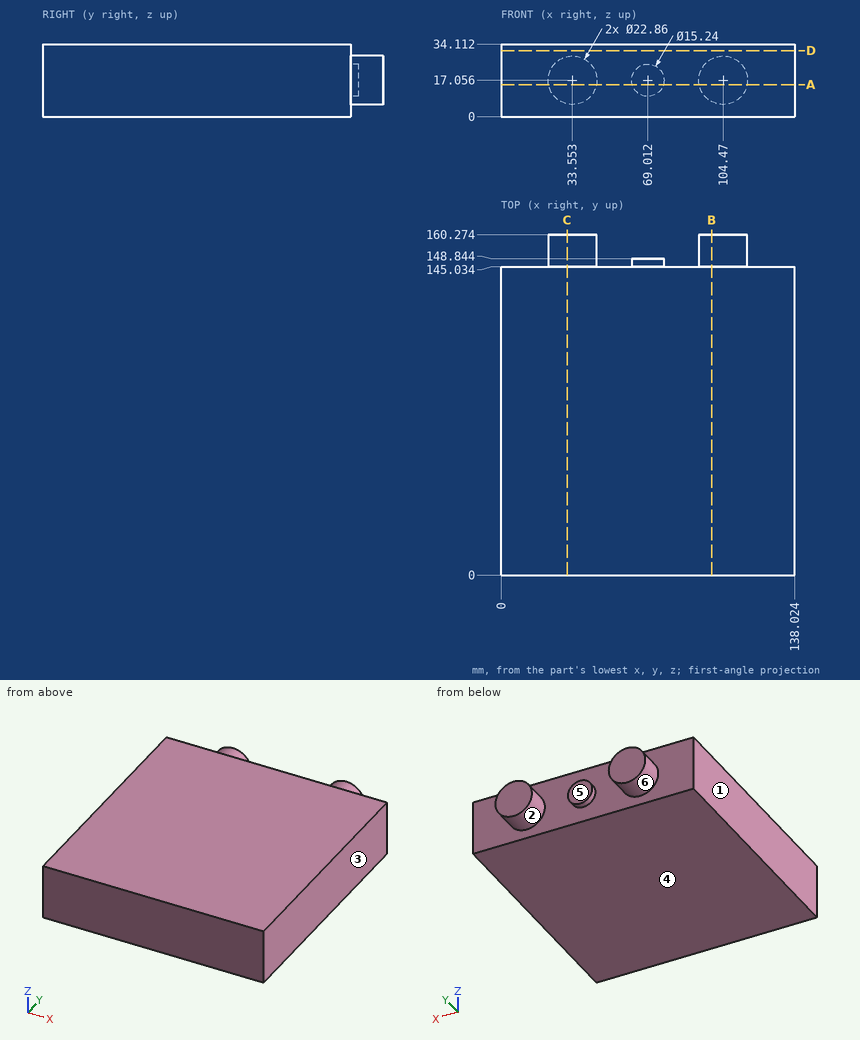
Could you check a few things on this drawing? It's one solid part, dimensions in mm from its lowest x, y, z. A direction names the side the tool comes from. Give positions to 0.01 mm unless a question says otherwise; leave off trailing zeros. Loops run counter-clockwise (first coordinate to the right, second up) from the corner with the lowest first, then second, coordinate; pieces in that order, holes last. Notation, with made-up numbers: M 49.5,-11.5 L 63.5,-11.5 A16 ccw 63.5,4.5 Z; hole C 79,-27.5 d10. An arc over 180 degrees is marked long. One line per question, with ' | ' between items. Start each with the question number.
Q1. If we section it at B-B (x = 99): Please give me the cut outline in (y, z).
Q2. If we section it at D-D (z = 31): Please give me the cut outline in (x, y).
Q3. If we mould it in two halves opening along X, with no side actions, what happens to the marked faces 1, 2 and 3? For each: +X half, -X half, draft (parallel to the pull), parting line (faces both ways), or undercut.
Q4. For the marked faces 4, 5 and 6, which set-ups out of +Z, -Z, +X, -X, +Y, -Y let a thin tool reach every point of the face, with its end or its side?
Q5. If we section it at A-A (z = 15): Please give me the cut outline in (x, y) (1 decimal), plus the area to 3 significant figures.
Q6. If I drill on line 1 (Y direction, x = 108.5, z = 29.5); line 2 (X direction, y = 152, z = 27) (1 decimal); line 3 (Z direction, x = 41.5, y = 153), over which ranges is the centre line in solid material (lowest first)? Write a range as from..to.
Q7. If we section it at C-C (x = 31): Please give me the cut outline in (y, z) (1 decimal), plus the area to 3 significant figures.
Q8. For pin 1 Ø10 at (x, z) = (56, 16.5) entering from +Y; pin 2 Ø7.5 at (x, z) = (65.5, 18.5) entering from +Y, each with a flat end and sliding along its axis, tell me the tip position at first contact or that it passes through.
Computed:
1) outline: M 0,0 L 145.03,0 L 145.03,7.02 L 160.27,7.02 L 160.27,27.09 L 145.03,27.09 L 145.03,34.11 L 0,34.11 Z
2) outline: M 0,0 L 138.02,0 L 138.02,145.03 L 0,145.03 Z
3) face 1: -X half | face 2: undercut | face 3: +X half
4) face 4: -Z, +X, -X, +Y, -Y | face 5: +Z, -Z, +Y | face 6: +Y
5) outline: M 0,0 L 138,0 L 138,145 L 115.7,145 L 115.7,160.3 L 93.2,160.3 L 93.2,145 L 76.3,145 L 76.3,148.8 L 61.7,148.8 L 61.7,145 L 44.8,145 L 44.8,160.3 L 22.3,160.3 L 22.3,145 L 0,145 Z | area: 20,800 mm²
6) line 1: y = 0..145.03 | line 2: x = 27.9..39.2, 98.8..110.1 | line 3: z = 8.84..25.27
7) outline: M 0,0 L 145,0 L 145,5.9 L 160.3,5.9 L 160.3,28.2 L 145,28.2 L 145,34.1 L 0,34.1 Z | area: 5,290 mm²
8) pin 1: stops at y = 145.03 | pin 2: stops at y = 148.84
